Design review of the part built by this model. Coordinates are the model's own, in mm. Face numbers are marked on the shaded views. A direction names the side the tool comes from. Coordinates: 2 decimals unless noted, no trailing zeros. Loops run counter-clockwise (first coordinate to the right, second up) from the corner with the lowest first, then second, coordinate; pieces in that order, holes last. Notation, with made-up numbers: (-31.5, -10) - (23.5, -10) arc R25 cw to (23.5, 15) - close; hole circle Ø6 at (4.5, 83). An arc over 180 degrees is marked (long way). One line per question, with ' | ' between items.
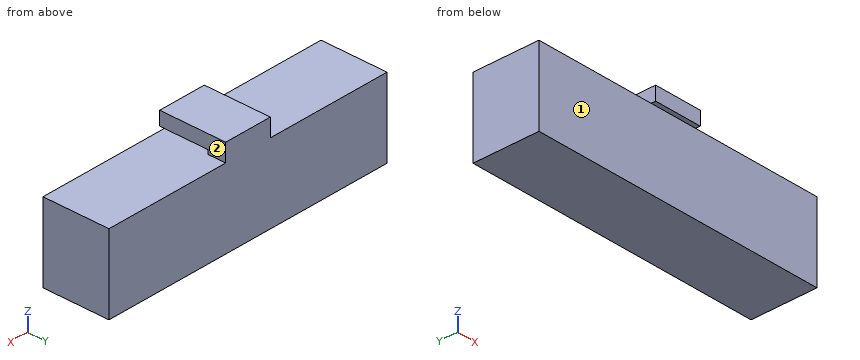
from build123d import *

# Parameters (mm, degrees)
ESQUISSE1_W             = 21.8
ESQUISSE1_H             = 4.8
BOSS_EXTRU_1_DEPTH      = 7
ESQUISSE2_W             = 9.15
ESQUISSE2_H             = 4.8
ENL_V_MAT_EXTRU_1_DEPTH = 1.3
ESQUISSE3_W             = 3.5
ESQUISSE3_H             = 0.3
ENL_V_MAT_EXTRU_2_DEPTH = 3.5


with BuildPart() as part:
    # Esquisse1 → Boss.-Extru.1 (new body)
    with BuildSketch(Plane.XY):
        Rectangle(ESQUISSE1_W, ESQUISSE1_H)
    extrude(amount=BOSS_EXTRU_1_DEPTH)

    # Esquisse2 → Enlèv. mat.-Extru.1 (cut)
    with BuildSketch(Plane.XY.offset(7)):
        with Locations((-6.325, 0)):
            Rectangle(ESQUISSE2_W, ESQUISSE2_H)
        with Locations((6.325, 0)):
            Rectangle(ESQUISSE2_W, ESQUISSE2_H)
    extrude(amount=-ENL_V_MAT_EXTRU_1_DEPTH, mode=Mode.SUBTRACT)

    # Esquisse3 → Enlèv. mat.-Extru.2 (cut)
    with BuildSketch(Plane.XZ.offset(2.4)):
        with Locations((0, 5.85)):
            Rectangle(ESQUISSE3_W, ESQUISSE3_H)
    extrude(amount=-ENL_V_MAT_EXTRU_2_DEPTH, mode=Mode.SUBTRACT)


solid = part.part
Q1. Take a section at B-B (x = 0.25). Give the boundary of the cut face in (y, z), plus the area to 4 significant figures.
Returned:
outline: (-2.4, 0) - (2.4, 0) - (2.4, 7) - (-2.4, 7) - (-2.4, 6) - (1.1, 6) - (1.1, 5.7) - (-2.4, 5.7) - close | area: 32.55 mm²
Q2. Take a section at D-D (x = 4.25). Give the boundary of the cut face in (y, z).
Returned:
outline: (-2.4, 0) - (2.4, 0) - (2.4, 5.7) - (-2.4, 5.7) - close
Q3. For pin 1 (0.7 mm diameter, centred on y = -1, z = 6.5, fed in from +X); pin 2 (1.4 mm diameter, centred on y = -1, z = 6.5, fed in from -X); pin 3 (2 mm diameter, centred on x = 8, y = -1, fed in from +Z), all flat-tipped, find the tip position at first contact; note any pin that passes through.
Returned:
pin 1: stops at x = 1.75 | pin 2: stops at x = -1.75 | pin 3: stops at z = 5.7
Q4. To check wall thickness, follow line 1 along Z through (x, y) = (-0.5, -0.35); line 2 along Z through (x, y) = (2, 1.15). State the ranges of each line that lie inside material, in increasing order.
Returned:
line 1: z = 0 to 5.7, 6 to 7 | line 2: z = 0 to 5.7
Q5. Take a section at C-C (y = 1.85). Give the boundary of the cut face in (x, z), plus the area to 3 significant figures.
Returned:
outline: (-10.9, 0) - (10.9, 0) - (10.9, 5.7) - (1.75, 5.7) - (1.75, 7) - (-1.75, 7) - (-1.75, 5.7) - (-10.9, 5.7) - close | area: 129 mm²
Q6. Tool access review of the marked faces 1 and 2: name each direction out of +Z, -Z, +X, -X, +Y, -Y from which nothing blocks a thin tool from reaching the whole face with its end or side.
Returned:
face 1: +Z, -Z, +X, -X, -Y | face 2: +Z, +X, +Y, -Y
Q7. Take a section at A-A (y = 0.8). Give the boundary of the cut face in (x, z).
Returned:
outline: (-10.9, 0) - (10.9, 0) - (10.9, 5.7) - (-10.9, 5.7) - close; (-1.75, 6) - (1.75, 6) - (1.75, 7) - (-1.75, 7) - close
